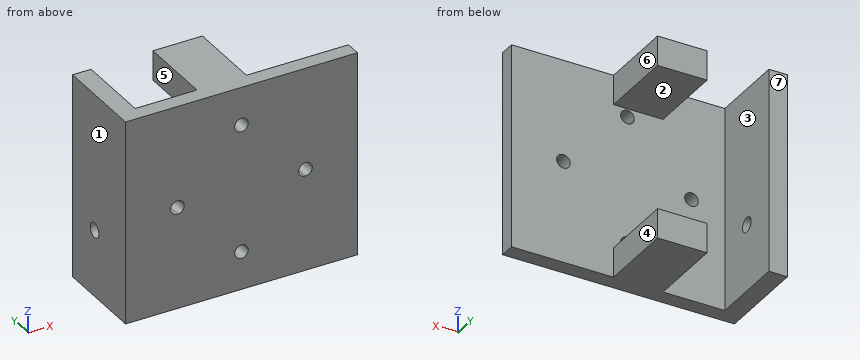
from build123d import *

# Parameters (mm, degrees)
SKIZZE1_W                       = 37.5
SKIZZE1_H                       = 33
AUFSATZ_LINEAR_AUSTRAGEN1_DEPTH = 2.5
SKIZZE2_W                       = 3
SKIZZE2_H                       = 33
SKIZZE2_W_2                     = 8
SKIZZE2_H_2                     = 4.8
AUFSATZ_LINEAR_AUSTRAGEN2_DEPTH = 12.3
SCHNITT_LINEAR_AUSTRAGEN3_DEPTH = 30.031922086
SKIZZE5_R                       = 1.2
SCHNITT_LINEAR_AUSTRAGEN4_DEPTH = 42.006584837


with BuildPart() as part:
    # Skizze1 → Aufsatz-Linear austragen1 (new body)
    with BuildSketch(Plane(origin=(0, 0, 0), x_dir=(1, 0, 0), z_dir=(0, 1, 0))):
        Rectangle(SKIZZE1_W, SKIZZE1_H)
    extrude(amount=AUFSATZ_LINEAR_AUSTRAGEN1_DEPTH)

    # Skizze2 → Aufsatz-Linear austragen2 (add)
    with BuildSketch(Plane(origin=(0, 2.5, 0), x_dir=(1, 0, 0), z_dir=(0, 1, 0))):
        with Locations((-17.25, 0)):
            Rectangle(SKIZZE2_W, SKIZZE2_H)
        with Locations((-1.75, -14.1)):
            Rectangle(SKIZZE2_W_2, SKIZZE2_H_2)
        with Locations((-1.75, 14.1)):
            Rectangle(SKIZZE2_W_2, SKIZZE2_H_2)
    extrude(amount=AUFSATZ_LINEAR_AUSTRAGEN2_DEPTH)

    # Skizze6 → Schnitt-Linear austragen3 (cut, through all)
    with BuildSketch(Plane.XZ):
        with BuildLine():
            ThreePointArc((-10.291545894, -1.098445774), (-9.551783389, -0.756868708), (-9.25, 0))
            ThreePointArc((-9.25, 0), (-9.551783389, 0.756868708), (-10.291545894, 1.098445774))
            ThreePointArc((-10.291545894, 1.098445774), (-10.35, 0), (-10.291545894, -1.098445774))
        make_face()
        with BuildLine():
            ThreePointArc((-10.291545894, -1.098445774), (-10.35, 0), (-10.291545894, 1.098445774))
            ThreePointArc((-10.291545894, 1.098445774), (-11.45, 0), (-10.291545894, -1.098445774))
        make_face()
        with BuildLine():
            ThreePointArc((-1.098445774, 10.291545894), (0, 9.25), (1.098445774, 10.291545894))
            ThreePointArc((1.098445774, 10.291545894), (0, 10.35), (-1.098445774, 10.291545894))
        make_face()
        with BuildLine():
            ThreePointArc((-1.098445774, 10.291545894), (0, 10.35), (1.098445774, 10.291545894))
            ThreePointArc((1.098445774, 10.291545894), (1.099611375, 10.320762617), (1.1, 10.35))
            ThreePointArc((1.1, 10.35), (-0.029237383, 11.449611375), (-1.098445774, 10.291545894))
        make_face()
        with BuildLine():
            ThreePointArc((10.291545894, -1.098445774), (11.106868708, -0.798216611), (11.45, 0))
            ThreePointArc((11.45, 0), (11.106868708, 0.798216611), (10.291545894, 1.098445774))
            ThreePointArc((10.291545894, 1.098445774), (10.35, 0), (10.291545894, -1.098445774))
        make_face()
        with BuildLine():
            ThreePointArc((10.291545894, -1.098445774), (10.35, 0), (10.291545894, 1.098445774))
            ThreePointArc((10.291545894, 1.098445774), (9.25, 0), (10.291545894, -1.098445774))
        make_face()
        with BuildLine():
            ThreePointArc((-1.098445774, -10.291545894), (-0.029237383, -11.449611375), (1.1, -10.35))
            ThreePointArc((1.1, -10.35), (1.099611375, -10.320762617), (1.098445774, -10.291545894))
            ThreePointArc((1.098445774, -10.291545894), (0, -10.35), (-1.098445774, -10.291545894))
        make_face()
        with BuildLine():
            ThreePointArc((-1.098445774, -10.291545894), (0, -10.35), (1.098445774, -10.291545894))
            ThreePointArc((1.098445774, -10.291545894), (0, -9.25), (-1.098445774, -10.291545894))
        make_face()
    extrude(amount=-SCHNITT_LINEAR_AUSTRAGEN3_DEPTH, mode=Mode.SUBTRACT)

    # Skizze5 → Schnitt-Linear austragen4 (cut, through all)
    with BuildSketch(Plane(origin=(-15.75, 0, 0), x_dir=(0, 0, -1), z_dir=(1, 0, 0))):
        with Locations((5.7, 8.65)):
            Circle(SKIZZE5_R)
    extrude(amount=-SCHNITT_LINEAR_AUSTRAGEN4_DEPTH, mode=Mode.SUBTRACT)


solid = part.part
The listing builds one solid part. Answer for the finished solid, in the listing's coordinates (mm). Face numbers are marked on the shaded views. A direction names the side the tool comes from. Give positions to 0.01 mm unless a question says otherwise; leave off trailing zeros. Write each loop counter-clockwise with the first axis right and the second up, starting at its lowest first coordinate (ties: lowest second). Pieces come first, ordered by that corner, then holes.
Item 1: Find the intervals of material crossed by line 1 along Y through (x, z) = (-16.6, -5.7); line 2 along X through (y, z) = (6.5, 12); line 3 along Z through (x, y) = (-0.5, 2), in increasing order.
Item 2: Flat-ended cylindrical pins translate along their axes: P1, Ø10, axis at x = 11.5, z = -0.5, coming from the +Y side; P2, Ø5.5, axis at y = 7, z = 14.5, coming from the +X side; P3, Ø4, axis at y = 8.65, z = -5.7, coming from the +X side. Find the tip coordinate at first contact, or state that the pin passes through.
Item 3: Section C-C, the plane x = 14.5 is taken. Write down the section's boundary in (y, z).
Item 4: Which of the six approach directions +Z, -Z, +X, -X, +Y, -Y give full straight-line access (tool end or side, diameter ignored) to the marked faces 5, 6 and 7?
Item 5: Section A-A, the plane y = 4.5 is taken. Write down the section's boundary in (x, z).
Item 6: Section B-B, the plane z = 3.5 is taken. Write down the section's boundary in (x, y).
Item 7: Determine the mould class of the marked faces 1, 2, 3 and 4 for opening direction X: released by +X, released by -X, zero draft, split by the parting line, or undercut.
Completed:
1. line 1: y = 0 to 7.45, 9.85 to 14.8
1. line 2: x = -18.75 to -15.75, -5.75 to 2.25
1. line 3: z = -16.5 to -11.33, -9.37 to 9.37, 11.33 to 16.5
2. P1: stops at y = 2.5
2. P2: stops at x = 2.25
2. P3: stops at x = -15.75
3. outline: (0, -16.5) - (2.5, -16.5) - (2.5, 16.5) - (0, 16.5) - close
4. face 5: +Z, -Z, +Y
4. face 6: +Z, -Z, +X, +Y
4. face 7: +Z, -Z, +X, -X, +Y
5. outline: (-18.75, -16.5) - (-15.75, -16.5) - (-15.75, 16.5) - (-18.75, 16.5) - close; (-5.75, -16.5) - (2.25, -16.5) - (2.25, -11.7) - (-5.75, -11.7) - close; (-5.75, 11.7) - (2.25, 11.7) - (2.25, 16.5) - (-5.75, 16.5) - close
6. outline: (-18.75, 0) - (18.75, 0) - (18.75, 2.5) - (-15.75, 2.5) - (-15.75, 14.8) - (-18.75, 14.8) - close
7. face 1: released by -X
7. face 2: zero draft
7. face 3: undercut
7. face 4: released by +X
